from build123d import *

# Parameters (mm, degrees)
F0_R     = 7.5
F1_DEPTH = 2
F3_DEPTH = 2
F5_DEPTH = 1


with BuildPart() as f1:
    # F0 (on Top) → F1 (new body)
    with BuildSketch(Plane.XY):
        Circle(F0_R)
    extrude(amount=F1_DEPTH)

    # F2 (on face) → F3 (join)
    with BuildSketch(Plane.XY.offset(2)):
        with BuildLine():
            ThreePointArc((-4.359569, -0.5816), (-4.048866, -2.485422), (-3.201723, -4.21846))
            ThreePointArc((-3.201723, -4.21846), (-1.763517, -5.989849), (0.471135, -6.450916))
            ThreePointArc((0.471135, -6.450916), (2.104993, -5.542203), (3.85862, -4.894092))
            ThreePointArc((3.85862, -4.894092), (5.530357, -3.673758), (5.763789, -1.6172))
            ThreePointArc((5.763789, -1.6172), (4.99478, 1.033842), (4.484988, 3.746685))
            ThreePointArc((4.484988, 3.746685), (4.307559, 2.089188), (4.484988, 0.43169))
            ThreePointArc((4.484988, 0.43169), (4.433756, -0.548224), (3.829129, -1.321065))
            ThreePointArc((3.829129, -1.321065), (3.396288, -0.731371), (3.409992, 0))
            ThreePointArc((3.409992, 0), (3.601771, 1.796582), (2.577243, 3.284811))
            ThreePointArc((2.577243, 3.284811), (1.342352, 4.895456), (1.246507, 6.922756))
            ThreePointArc((1.246507, 6.922756), (0.746139, 4.772952), (1.246507, 2.623147))
            ThreePointArc((1.246507, 2.623147), (1.445906, 1.76644), (1.246507, 0.909734))
            ThreePointArc((1.246507, 0.909734), (0.802459, 1.438025), (0.558072, 2.083429))
            ThreePointArc((0.558072, 2.083429), (-0.141358, 4.191438), (-1.347645, 6.056319))
            ThreePointArc((-1.347645, 6.056319), (-0.903638, 4.8169), (-0.814198, 3.503393))
            ThreePointArc((-0.814198, 3.503393), (-1.023492, 1.611686), (-1.718377, -0.160176))
            ThreePointArc((-1.718377, -0.160176), (-2.008384, -0.350929), (-2.2774, -0.570297))
            ThreePointArc((-2.2774, -0.570297), (-3.112946, 0.306997), (-3.216468, 1.514086))
            ThreePointArc((-3.216468, 1.514086), (-2.859593, 2.940059), (-2.873537, 4.409944))
            ThreePointArc((-2.873537, 4.409944), (-3.321426, 3.190102), (-3.864225, 2.00943))
            ThreePointArc((-3.864225, 2.00943), (-4.340752, 0.757667), (-4.359569, -0.5816))
        make_face()
    extrude(amount=F3_DEPTH)

    # F4 (on face) → F5 (join)
    with BuildSketch(Plane.XY.offset(4)):
        with BuildLine():
            ThreePointArc((-2.683389, -2.667802), (-2.380518, -3.229598), (-2.075762, -3.790374))
            ThreePointArc((-2.075762, -3.790374), (-0.413473, -5.59377), (1.818095, -4.576151))
            ThreePointArc((1.818095, -4.576151), (2.259919, -4.381156), (2.73005, -4.270664))
            ThreePointArc((2.73005, -4.270664), (4.260916, -3.418142), (4.605096, -1.700036))
            ThreePointArc((4.605096, -1.700036), (3.983593, -2.740688), (2.789322, -2.947901))
            ThreePointArc((2.789322, -2.947901), (2.209801, -2.674705), (2.119534, -2.040409))
            ThreePointArc((2.119534, -2.040409), (2.35368, -0.297977), (1.824975, 1.378736))
            ThreePointArc((1.824975, 1.378736), (1.702683, -0.046192), (1.038666, -1.312863))
            ThreePointArc((1.038666, -1.312863), (0.529939, -1.321844), (0.403569, -0.82898))
            ThreePointArc((0.403569, -0.82898), (0.176498, 0.455843), (-0.564196, 1.529949))
            ThreePointArc((-0.564196, 1.529949), (-0.457664, -0.055376), (-0.789172, -1.609308))
            ThreePointArc((-0.789172, -1.609308), (-1.448975, -1.733967), (-2.108778, -1.609308))
            ThreePointArc((-2.108778, -1.609308), (-2.701327, -1.433486), (-3.197515, -1.06494))
            ThreePointArc((-3.197515, -1.06494), (-3.086289, -1.913149), (-2.683389, -2.667802))
        make_face()
    extrude(amount=F5_DEPTH)


solid = f1.part
Could you check a few things on this model? Use its own coordinates, in mm. A direction names the side the tool comes from. Coordinates: 2 decimals unless noted, no trailing zeros. Order: outer loops, then holes, each group sorted by start corner. A loop starts at its lowest first (then second) coordinate and runs counter-clockwise, first axis right, second up.
Q1. Thinking about a two-plate mould opening in X: for faces 5 (the cylindrical face through (4.308, 2.113, 2.986)), 6 (the cylindrical face through (-3.314, 3.207, 2.986)), 7 (the cylindrical face through (4.246, -3.439, 4.493)), which applies, released by +X, released by -X, zero draft, split by the parting line, or undercut?
Q2. Suppose I cut it at C-C on x = 0. Please give me the cut outline in (y, z).
Q3. Please list where these lines run through material, in increasing order: L1, parallel to Z at x = -3.25, y = -6; L2, parallel to Z at x = -1.25, y = -6; L3, parallel to X at y = 3, z = 3.45.
Q4. Suppose I cut it at A-A on z = 3. Please give me the cut outline in (x, y), and give its area (3 significant figures).
Q5. Suppose I cut it at D-D on z = 0.95. Please give me the cut outline in (x, y).
Q6. Which directions (+Z, -Z, +X, -X, +Y, -Y) give clear straight access to the entire face, cutting with the end or side of a thin tool? Please do faces 1 (the cylindrical face through (-4.057, -2.46, 2.986)), 2 (the cylindrical face through (2.081, -5.553, 2.986)), 3 (the cylindrical face through (5.515, -3.699, 2.986)), 4 (the cylindrical face through (-3.106, 0.291, 2.986)).
Q7. Will these pins go through, and if not, where does the flat tip stop? pin 1 (3 mm diameter, centred on x = -1.5, z = 4.5, fed in from +Y); pin 2 (2 mm diameter, centred on x = -4.5, z = 1, fed in from +Y).
Q8. Suppose I cut it at B-B on x = 5.5. Please give me the cut outline in (y, z), and give its area (3 significant figures).
Answer:
1. face 5: undercut
1. face 6: released by -X
1. face 7: released by +X
2. outline: (-7.5, 0) - (7.5, 0) - (7.5, 2) - (3.88, 2) - (3.88, 4) - (0.82, 4) - (0.82, 5) - (-5.64, 5) - (-5.64, 4) - (-6.48, 4) - (-6.48, 2) - (-7.5, 2) - close
3. L1: z = 0 to 2
3. L2: z = 0 to 4
3. L3: x = -3.4 to -2.85, -0.82 to 0.33, 1.08 to 2.92, 4.36 to 4.6
4. outline: (-4.36, -0.58) arc R6.61 ccw to (-3.2, -4.22) arc R3.4 ccw to (0.47, -6.45) arc R12.19 cw to (3.86, -4.89) arc R2.57 ccw to (5.76, -1.62) arc R28.59 cw to (4.48, 3.75) arc R7.83 ccw to (4.48, 0.43) arc R1.63 cw to (3.83, -1.32) arc R1.14 cw to (3.41, 0) arc R2.6 ccw to (2.58, 3.28) arc R3.4 cw to (1.25, 6.92) arc R4.87 ccw to (1.25, 2.62) arc R1.94 cw to (1.25, 0.91) arc R2.06 cw to (0.56, 2.08) arc R8.78 ccw to (-1.35, 6.06) arc R4.79 cw to (-0.81, 3.5) arc R7.24 cw to (-1.72, -0.16) arc R3.4 ccw to (-2.28, -0.57) arc R1.83 cw to (-3.22, 1.51) arc R5.79 ccw to (-2.87, 4.41) arc R16.45 cw to (-3.86, 2.01) arc R3.85 ccw to start
4. area: 72.3 mm2
5. outline: circle Ø15 at (0, 0)
6. face 1: +Z, -X, -Y
6. face 2: +Z, +X, -Y
6. face 3: +Z, +X
6. face 4: +Z
7. pin 1: stops at y = 6.06
7. pin 2: stops at y = 6.63
8. outline: (-5.1, 0) - (5.1, 0) - (5.1, 2) - (-0.81, 2) - (-0.81, 4) - (-3.72, 4) - (-3.72, 2) - (-5.1, 2) - close
8. area: 26.2 mm2
